```python
from build123d import *

# Parameters (mm, degrees)
F0_W     = 0.254
F0_H     = 17.78
F0_R     = 6.35
F0_R_2   = 1.4224
F1_DEPTH = 3.175


with BuildPart() as f1:
    # F0 (on Top) → F1 (new body)
    with BuildSketch(Plane.XY):
        with BuildLine():
            Line((63.5, 0), (63.5, 88.9))
            Line((63.5, 88.9), (-63.5, 88.9))
            Line((-63.5, 88.9), (-63.5, 0))
            Line((-63.5, 0), (-63.5, -8.594495))
            ThreePointArc((-63.5, -8.594495), (0, -67.942486), (63.5, -8.594495))
            Line((63.5, -8.594495), (63.5, 0))
        make_face()
        with Locations((-23.6855, -29.842486)):
            Rectangle(F0_W, F0_H, mode=Mode.SUBTRACT)
        with Locations((-36.2585, -10.325997)):
            Circle(F0_R, mode=Mode.SUBTRACT)
        with Locations((-40.64, 5.08)):
            Circle(F0_R_2, mode=Mode.SUBTRACT)
        with Locations((23.9395, -29.842486)):
            Rectangle(F0_W, F0_H, mode=Mode.SUBTRACT)
        with Locations((36.7665, -9.239232)):
            Circle(F0_R, mode=Mode.SUBTRACT)
        with Locations((40.64, 5.08)):
            Circle(F0_R_2, mode=Mode.SUBTRACT)
        with Locations((-57.15, 17.4498)):
            Circle(F0_R_2, mode=Mode.SUBTRACT)
        with Locations((-57.15, 50.8)):
            Circle(F0_R_2, mode=Mode.SUBTRACT)
        with Locations((-40.64, 76.2)):
            Circle(F0_R_2, mode=Mode.SUBTRACT)
        with Locations((57.15, 17.4498)):
            Circle(F0_R_2, mode=Mode.SUBTRACT)
        with Locations((57.15, 50.8)):
            Circle(F0_R_2, mode=Mode.SUBTRACT)
        with Locations((40.64, 76.2)):
            Circle(F0_R_2, mode=Mode.SUBTRACT)
        with BuildLine():
            ThreePointArc((63.5, -8.594495), (63.645238, -4.297248), (63.5, 0))
            Line((63.5, 0), (63.5, -8.594495))
        make_face()
        with BuildLine():
            Line((-63.5, -8.594495), (-63.5, 0))
            ThreePointArc((-63.5, 0), (-63.645238, -4.297248), (-63.5, -8.594495))
        make_face()
    extrude(amount=F1_DEPTH)


solid = f1.part
```
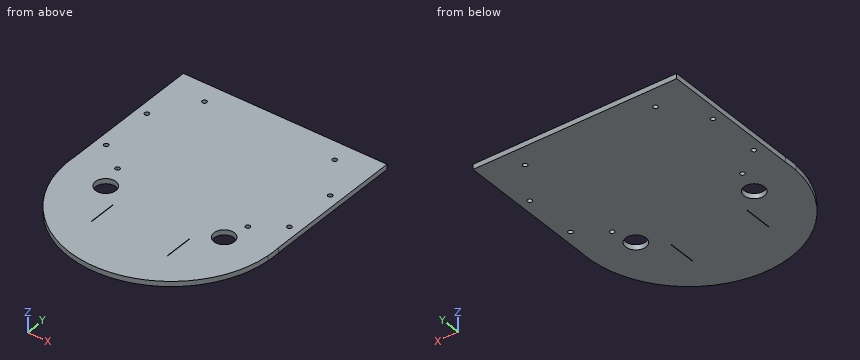
Model file for the job. Use its own axes, mm. Give positions to 0.01 mm unless a question says otherwise; leave off trailing zeros. Write each loop counter-clockwise with the first axis right and the second up, starting at its lowest first coordinate (ties: lowest second). Pieces come first, ordered by that corner, then holes. Notation, with made-up numbers: M 70.25,-14.75 L 126.25,-14.75 A17 ccw 126.25,8.25 Z; hole C -1.75,14.25 d2. An arc over 180 degrees is marked long. Use a Markdown table: item, result.
1) Cut at D-D (x = 49). List the corners of the cut face in (y, z) (3 decimals).
Responses:
| item | result |
|---|---|
| outline | M -44.914,0 L 88.9,0 L 88.9,3.175 L -44.914,3.175 Z |
2) Cut at C-C (y = -6). List the corners of the cut face in (x, z) (3 decimals), and give its area (3 significant figures).
Responses:
| item | result |
|---|---|
| outline | M -63.622,0 L -40.907,0 L -40.907,3.175 L -63.622,3.175 Z; M -31.61,0 L 31.305,0 L 31.305,3.175 L -31.61,3.175 Z; M 42.228,0 L 63.622,0 L 63.622,3.175 L 42.228,3.175 Z |
| area | 340 mm2 |
3) Pin check, flat tips, straight feed: pin 1 (1.6 mm diameter, centred on y = 46.5, z = 2, fed in from +X); pin 2 (1 mm diameter, centred on y = -32, z = 2, fed in from +X); pin 3 (10 mm diameter, centred on x = -36.26, y = -10.33, fed in from +Z). Stop position of each tip, or through.
Responses:
| item | result |
|---|---|
| pin 1 | stops at x = 63.5 |
| pin 2 | stops at x = 57.54 |
| pin 3 | passes through |
4) Cut at B-B (z = 1.8). Give the number of separate pieces and of enclosed holes in the cut face, and give its area (3 significant figures).
Responses:
| item | result |
|---|---|
| separate pieces | 1 |
| enclosed holes | 12 |
| area | 17,900 mm2 |
5) Cut at A-A (y = -29). List the corners of the cut face in (x, z) (1 decimal).
Responses:
| item | result |
|---|---|
| outline | M -58.7,0 L -23.8,0 L -23.8,3.2 L -58.7,3.2 Z; M -23.6,0 L 23.8,0 L 23.8,3.2 L -23.6,3.2 Z; M 24.1,0 L 58.7,0 L 58.7,3.2 L 24.1,3.2 Z |
6) Drill centre lines: line 1 (X direction, y = 76.2, z = 2.3); line 2 (Y direction, x = 57.15, z = 1.4); line 3 (Y direction, x = 40.64, z = 2.35). Where is each one in solid material? Low to high. Write a range as from..to.
Responses:
| item | result |
|---|---|
| line 1 | x = -63.5..-42.06, -39.22..39.22, 42.06..63.5 |
| line 2 | y = -32.31..16.03, 18.87..49.38, 52.22..88.9 |
| line 3 | y = -53.28..-14.27, -4.21..3.66, 6.5..74.78, 77.62..88.9 |
